Part model, mm, in its own coordinate system. Face numbers are marked on the shaded views. Coordinates: 2 decimals unless noted, no trailing zeros. Loops run counter-clockwise (first coordinate to the right, second up) from the corner with the lowest first, then second, coordinate; pieces in that order, holes last. Notation, with made-up numbers: (-2.75, 6) - (51.25, 6) arc R28 cw to (51.25, 31) - close; hole circle Ø5 at (55.5, 21.5). An arc over 180 degrees is marked (long way). Use a Markdown table: item, result. Add a question column.
1. Band-saw the part on A-A, the plane y = -17.7. Give the cut face in (x, z), plus the area to 3 significant figures.
2. Pull direction Y, two halves, no side cores. Call the marked faces 1, 2 and 3: pulls with the +Y half, pulls with the -Y half, needs draft (parallel to the pull), parting line crosses it, or undercut.
3. Band-saw the part on C-C, the plane x = -59. Give the cut face in (y, z).
4. Drop flat-ended pins along their axis: pin 1 (4 mm diameter, centred on y = -11, z = 1, fed in from +X); pin 2 (1 mm diameter, centred on x = -50, z = 5, fed in from -Y); pin 3 (3 mm diameter, centred on x = -63.5, y = 42, fed in from -Z); pin 4 (1.5 mm diameter, centred on x = -52, z = 5, fed in from -Y). Give the stop position or say it passes through.
5. Band-saw the part on D-D, the plane y = 4. Give the cut face in (x, z), plus the area to 3 significant figures.
6. Band-saw the part on B-B, the plane z = 6. Give the cut face in (x, y).
7. Wall check: probe 1 along Y at (x, z) = (-47, 2.25); probe 2 along Y at (x, z) = (-46.5, 7); probe 3 along X at (y, z) = (-13, 4.25). Give the ranges that are in metal, low to high. Write a range as [from, to].
from build123d import *

# Parameters (mm, degrees)
CROQUIS1_R              = 2.1
SALIENTE_EXTRUIR1_DEPTH = 10


with BuildPart() as part:
    # Croquis1 → Saliente-Extruir1 (new body)
    with BuildSketch(Plane.XY):
        with BuildLine():
            Line((-43.685266481, -9.509101851), (-55.484948694, 13.222697812))
            ThreePointArc((-55.484948694, 13.222697812), (-56.263095716, 15.220767285), (-56.597387965, 17.338795401))
            Line((-56.597387965, 17.338795401), (-57.734092582, 40.460761941))
            ThreePointArc((-57.734092582, 40.460761941), (-57.592357435, 41.912848633), (-57.037475041, 43.262200381))
            ThreePointArc((-57.037475041, 43.262200381), (-63.397480334, 53.832057006), (-68.690069236, 42.689344629))
            ThreePointArc((-68.690069236, 42.689344629), (-68.005510605, 41.40092523), (-67.722030303, 39.969742507))
            Line((-67.722030303, 39.969742507), (-66.478182752, 14.668357223))
            ThreePointArc((-66.478182752, 14.668357223), (-66.143890502, 12.550329107), (-65.365743481, 10.552259633))
            Line((-65.365743481, 10.552259633), (-52.560764931, -14.116218874))
            ThreePointArc((-52.560764931, -14.116218874), (-52.084712706, -15.495355776), (-52.027049902, -16.95320327))
            ThreePointArc((-52.027049902, -16.95320327), (-41.842018175, -23.912848963), (-41.672301733, -11.578233615))
            ThreePointArc((-41.672301733, -11.578233615), (-42.831358598, -10.692100558), (-43.685266481, -9.509101851))
        make_face()
        with Locations((-45.067, -17.7)):
            Circle(CROQUIS1_R, mode=Mode.SUBTRACT)
        with Locations((-63.053766888, 46.840500594)):
            Circle(CROQUIS1_R, mode=Mode.SUBTRACT)
    extrude(amount=SALIENTE_EXTRUIR1_DEPTH)


solid = part.part
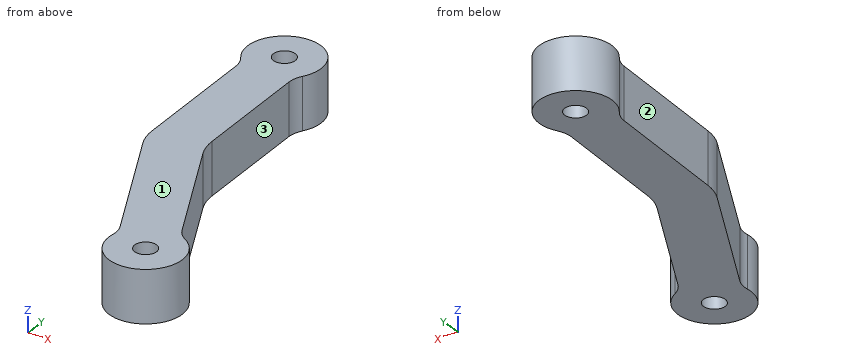
Geometry check:
| question | item | result |
|---|---|---|
| 1 | outline | (-52.07, 0) - (-47.17, 0) - (-47.17, 10) - (-52.07, 10) - close; (-42.97, 0) - (-38.07, 0) - (-38.07, 10) - (-42.97, 10) - close |
| 1 | area | 98.0 mm^2 |
| 2 | face 1 | needs draft |
| 2 | face 2 | pulls with the -Y half |
| 2 | face 3 | undercut |
| 3 | outline | (-1.71, 0) - (52.55, 0) - (52.55, 10) - (-1.71, 10) - close |
| 4 | pin 1 | stops at x = -39.88 |
| 4 | pin 2 | stops at y = -23.12 |
| 4 | pin 3 | stops at z = 0 |
| 4 | pin 4 | stops at y = -20.98 |
| 5 | outline | (-61.96, 0) - (-50.7, 0) - (-50.7, 10) - (-61.96, 10) - close |
| 5 | area | 113 mm^2 |
| 6 | outline | (-68.69, 42.69) arc R5 cw to (-67.72, 39.97) - (-66.48, 14.67) arc R10 ccw to (-65.37, 10.55) - (-52.56, -14.12) arc R5 cw to (-52.03, -16.95) arc R7 ccw (long way) to (-41.67, -11.58) arc R5 cw to (-43.69, -9.51) - (-55.48, 13.22) arc R10 cw to (-56.6, 17.34) - (-57.73, 40.46) arc R5 cw to (-57.04, 43.26) arc R7 ccw (long way) to start; hole circle Ø4.2 at (-63.05, 46.84); hole circle Ø4.2 at (-45.07, -17.7) |
| 7 | probe 1 | y = [-24.43, -18.52], [-16.88, -3.12] |
| 7 | probe 2 | y = [-24.55, -19.24], [-16.16, -4.09] |
| 7 | probe 3 | x = [-53.14, -39.88] |
